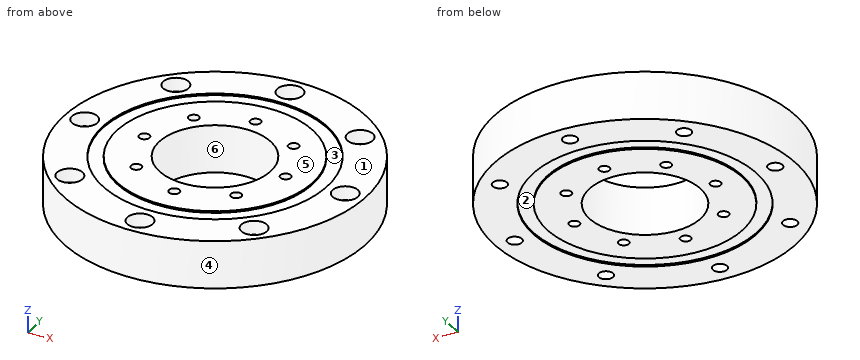
from build123d import *

# Parameters (mm, degrees)
SKETCH_1_R                   = 47.5
EXTRUDE_1_DEPTH              = 7.5
SKETCH_2_R                   = 17.5
CUT_EXTRUDE_1_DEPTH          = 16
SKETCH_3_R                   = 35.25
SKETCH_3_R_2                 = 30.75
CUT_EXTRUDE_2_DEPTH          = 0.5
HOLE_WIZARD_M4_1_D           = 4.5
HOLE_WIZARD_M4_1_CBORE_D     = 8
HOLE_WIZARD_M4_1_CBORE_DEPTH = 4.4
M4X0_7_1_D                   = 3.3
PATTERN_CIRCULAR_1_COUNT     = 8


with BuildPart() as part:
    # 草圖1 → 填料-伸長1 (new body, symmetric)
    with BuildSketch(Plane.XY):
        Circle(SKETCH_1_R)
    extrude(amount=EXTRUDE_1_DEPTH, both=True)

    # 草圖2 → 除料-伸長1 (cut, through all)
    with BuildSketch(Plane.XY.offset(7.5)):
        Circle(SKETCH_2_R)
    extrude(amount=-CUT_EXTRUDE_1_DEPTH, mode=Mode.SUBTRACT)

    # 草圖3 → 除料-伸長2 (cut)
    with BuildSketch(Plane.XY.offset(7.5)):
        Circle(SKETCH_3_R)
        Circle(SKETCH_3_R_2, mode=Mode.SUBTRACT)
    cut_extrude_2 = extrude(amount=-CUT_EXTRUDE_2_DEPTH, mode=Mode.SUBTRACT)

    # 鏡射1: 除料-伸長2 across plane
    add(cut_extrude_2.mirror(Plane.XY), mode=Mode.SUBTRACT)

    # M4 凹頭蓋螺釘的柱孔1 (through all)
    with Locations(Plane.XY.offset(7.5)):
        with Locations((0, 41.5)):
            hole_wizard_m4_1 = CounterBoreHole(HOLE_WIZARD_M4_1_D / 2, HOLE_WIZARD_M4_1_CBORE_D / 2, HOLE_WIZARD_M4_1_CBORE_DEPTH)

    # M4x0.7 螺紋孔1 (through all)
    with Locations(Plane.XY.offset(7.5)):
        with Locations((0, 22.5)):
            m4x0_7_1 = Hole(M4X0_7_1_D / 2)

    # 環狀複製排列1: M4 凹頭蓋螺釘的柱孔1, M4x0.7 螺紋孔1 ×8 about axis
    pattern_circular_1_axis = Axis((0, 0, 0), (0, 0, 1))
    for i in range(1, PATTERN_CIRCULAR_1_COUNT):
        add(hole_wizard_m4_1.rotate(pattern_circular_1_axis, i * 360 / PATTERN_CIRCULAR_1_COUNT), mode=Mode.SUBTRACT)
        add(m4x0_7_1.rotate(pattern_circular_1_axis, i * 360 / PATTERN_CIRCULAR_1_COUNT), mode=Mode.SUBTRACT)


solid = part.part
Model file for the job. Use its own axes, mm. Face numbers are marked on the shaded views. A direction names the side the tool comes from. Round coordinates to 2 decimals unless told otherwise and drop trailing zeros. Order: outer loops, then holes, each group sorted by start corner. A loop starts at its lowest first (then second) coordinate and runs counter-clockwise, first axis right, second up.
(1) Band-saw the part on B-B (y = -7). List the corners of the cut face in (x, z), then the cut area to 3 significant figures.
(2) Band-saw the part on A-A (x = 9.5). List the corners of the cut face in (y, z).
(3) Pin check, flat tips, straight feed: pin 1 (2.5 mm diameter, centred on x = -22.5, y = 0, fed in from -Z); pin 2 (3 mm diameter, centred on x = 6, y = -32.5, fed in from +Z); pin 3 (5 mm diameter, centred on x = 0, y = -41.5, fed in from +Z); pin 4 (6 mm diameter, centred on y = 34.5, z = -0.5, fed in from -X). Stop position of each tip, or through.
(4) Drill centre lines: line 1 (Y direction, x = 0, z = 4.25); line 2 (Y direction, x = 28.5, z = -6.25); line 3 (X direction, y = 26.5, z = 5.5). Where is each one in solid material? Low to high.
(5) 3-axis set-ups, long thin cutter, end or side, ignore diameter. For the marked faces 1, 2 and 3: which of +Z, -Z, +X, -X, +Y, -Y reach the whole face in a straight line?
(6) Pull direction Y, two halves, no side cores. Call the marked faces 4, 5 and 6: released by +Y, released by -Y, zero draft, split by the parting line, or undercut.
(7) Band-saw the part on C-C (z = 5.5). Give the number of separate pieces and of enclosed holes in the cut face, then the cut area to 3 significant figures.
Verdict:
1. outline: (-46.98, -7.5) - (-34.55, -7.5) - (-34.55, -7) - (-29.94, -7) - (-29.94, -7.5) - (-16.04, -7.5) - (-16.04, 7.5) - (-29.94, 7.5) - (-29.94, 7) - (-34.55, 7) - (-34.55, 7.5) - (-46.98, 7.5) - close; (16.04, -7.5) - (29.94, -7.5) - (29.94, -7) - (34.55, -7) - (34.55, -7.5) - (46.98, -7.5) - (46.98, 7.5) - (34.55, 7.5) - (34.55, 7) - (29.94, 7) - (29.94, 7.5) - (16.04, 7.5) - close
1. area: 919 mm2
2. outline: (-46.54, -7.5) - (-33.95, -7.5) - (-33.95, -7) - (-29.25, -7) - (-29.25, -7.5) - (-14.7, -7.5) - (-14.7, 7.5) - (-29.25, 7.5) - (-29.25, 7) - (-33.95, 7) - (-33.95, 7.5) - (-46.54, 7.5) - close; (14.7, -7.5) - (29.25, -7.5) - (29.25, -7) - (33.95, -7) - (33.95, -7.5) - (46.54, -7.5) - (46.54, 7.5) - (33.95, 7.5) - (33.95, 7) - (29.25, 7) - (29.25, 7.5) - (14.7, 7.5) - close
3. pin 1: passes through
3. pin 2: stops at z = 7
3. pin 3: stops at z = 3.1
3. pin 4: stops at x = -35.55
4. line 1: y = -47.5 to -45.5, -37.5 to -24.15, -20.85 to -17.5, 17.5 to 20.85, 24.15 to 37.5, 45.5 to 47.5
4. line 2: y = -38 to -31.43, -27.26 to 27.26, 31.43 to 38
4. line 3: x = -39.42 to -32.16, -26.53 to 26.53, 32.16 to 39.42
5. face 1: +Z, +X, -X, +Y, -Y
5. face 2: -Z
5. face 3: +Z
6. face 4: split by the parting line
6. face 5: zero draft
6. face 6: undercut
7. separate pieces: 1
7. enclosed holes: 17
7. area: 5,660 mm2
